from build123d import *

# Parameters (mm, degrees)
SKETCH1_W           = 20
SKETCH1_H           = 20
BOSS_EXTRUDE1_DEPTH = 20
SKETCH2_W           = 16.9
SKETCH2_H           = 16.9
BOSS_EXTRUDE2_DEPTH = 20
SKETCH3_W           = 16.9
SKETCH3_H           = 16.9
BOSS_EXTRUDE3_DEPTH = 20
SKETCH4_W           = 16.9
SKETCH4_H           = 16.9
BOSS_EXTRUDE4_DEPTH = 20


with BuildPart() as part:
    # Sketch1 → Boss-Extrude1 (new body)
    with BuildSketch(Plane(origin=(0, 0, 0), x_dir=(1, 0, 0), z_dir=(0, 1, 0))):
        Rectangle(SKETCH1_W, SKETCH1_H)
    extrude(amount=BOSS_EXTRUDE1_DEPTH)

    # Sketch2 → Boss-Extrude2 (add)
    with BuildSketch(Plane(origin=(0, 20, 0), x_dir=(1, 0, 0), z_dir=(0, 1, 0))):
        Rectangle(SKETCH2_W, SKETCH2_H)
    extrude(amount=BOSS_EXTRUDE2_DEPTH)

    # Sketch3 → Boss-Extrude3 (add)
    with BuildSketch(Plane(origin=(10, 0, 0), x_dir=(0, 0, -1), z_dir=(1, 0, 0))):
        with Locations((0, 10)):
            Rectangle(SKETCH3_W, SKETCH3_H)
    extrude(amount=BOSS_EXTRUDE3_DEPTH)

    # Sketch4 → Boss-Extrude4 (add)
    with BuildSketch(Plane(origin=(0, 0, -10), x_dir=(-1, 0, 0), z_dir=(0, 0, -1))):
        with Locations((0, 10)):
            Rectangle(SKETCH4_W, SKETCH4_H)
    extrude(amount=BOSS_EXTRUDE4_DEPTH)


solid = part.part
Could you check a few things on this model? Use its own coordinates, in mm. A direction names the side the tool comes from. Coordinates: 2 decimals unless noted, no trailing zeros. Order: outer loops, then holes, each group sorted by start corner. A loop starts at its lowest first (then second) coordinate and runs counter-clockwise, first axis right, second up.
Q1. Suppose I cut it at C-C on z = -27. Please give me the cut outline in (x, y), and give its area (3 significant figures).
Q2. Suppose I cut it at A-A on x = -1. Please give me the cut outline in (y, z).
Q3. Which directions (+Z, -Z, +X, -X, +Y, -Y) give clear straight access to the entire face, cutting with the end or side of a thin tool? Please do faces 1 (the flat face through (20, 10, 8.45)), 2 (the flat face through (0, 18.45, -20)), 3 (the flat face through (20, 10, -8.45)), 4 (the flat face through (-8.45, 30, 0)).
Q4. Please list where these lines run through material, in increasing order: L1, parallel to X at y = 28.5, z = 7; L2, parallel to Y at x = 7.5, z = -15; L3, parallel to X at y = 19, z = -4.
Q5. Suppose I cut it at D-D on x = 12.5. Please give me the cut outline in (y, z).
Q6. Suppose I cut it at B-B on y = 3. Please give me the cut outline in (x, z).
Q7. Will these pins go through, and if not, where does the flat tip stop? pin 1 (13.5 mm diameter, centred on x = -4, y = 31, fed in from -Z); pin 2 (5 mm diameter, centred on x = 24.5, z = -3.5, fed in from +Y); pin 3 (13.5 mm diameter, centred on x = 20, y = 8.5, fed in from +Z); pin 4 (6 mm diameter, centred on x = -2.5, z = 0, fed in from -Y).
Answer:
1. outline: (-8.45, 1.55) - (8.45, 1.55) - (8.45, 18.45) - (-8.45, 18.45) - close
1. area: 286 mm2
2. outline: (0, -10) - (1.55, -10) - (1.55, -30) - (18.45, -30) - (18.45, -10) - (20, -10) - (20, -8.45) - (40, -8.45) - (40, 8.45) - (20, 8.45) - (20, 10) - (0, 10) - close
3. face 1: +Z, +X, +Y, -Y
3. face 2: -Z, +X, -X, +Y
3. face 3: -Z, +X, +Y, -Y
3. face 4: +Z, -Z, -X, +Y
4. L1: x = -8.45 to 8.45
4. L2: y = 1.55 to 18.45
4. L3: x = -10 to 10
5. outline: (1.55, -8.45) - (18.45, -8.45) - (18.45, 8.45) - (1.55, 8.45) - close
6. outline: (-10, -10) - (-8.45, -10) - (-8.45, -30) - (8.45, -30) - (8.45, -10) - (10, -10) - (10, -8.45) - (30, -8.45) - (30, 8.45) - (10, 8.45) - (10, 10) - (-10, 10) - close
7. pin 1: stops at z = -8.45
7. pin 2: stops at y = 18.45
7. pin 3: stops at z = 8.45
7. pin 4: stops at y = 0
